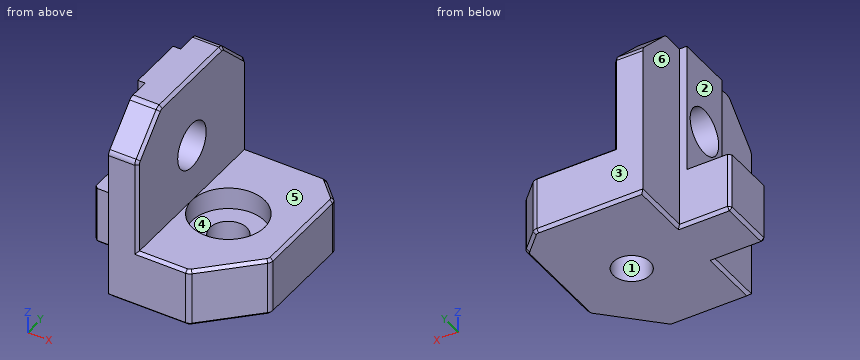
from build123d import *

# Parameters (mm, degrees)
CYLINDER014_R     = 3.15
CYLINDER014_DEPTH = 15
BOX016_W          = 4
BOX016_H          = 24
BOX016_DEPTH      = 26
CHAMFER024_SIZE   = 5
FILLET006_R       = 1
CHAMFER025_SIZE   = 0.4
CYLINDER012_R     = 2.525
CYLINDER012_DEPTH = 35
CYLINDER013_R     = 5
CYLINDER013_DEPTH = 5
BOX018_W          = 18
BOX018_H          = 24
BOX018_DEPTH      = 8
CHAMFER021_SIZE   = 7
CHAMFER022_SIZE   = 3
FILLET005_R       = 1
CHAMFER023_SIZE   = 0.4
BOX019_W          = 2
BOX019_H          = 7.8
BOX019_DEPTH      = 18
BOX017_W          = 8
BOX017_H          = 7.8
BOX017_DEPTH      = 8
CHAMFER026_SIZE   = 0.4


with BuildPart() as cylinder014:
    # Cylinder014 → Cylinder014 (new body)
    with BuildSketch(Plane(origin=(9, 15, 56), x_dir=(0, -1, 0), z_dir=(-1, 0, 0))):
        Circle(CYLINDER014_R)
    extrude(amount=CYLINDER014_DEPTH)


with BuildPart() as chamfer025:
    # Box016 → Box016 (new body)
    with BuildSketch(Plane(origin=(0, 3, 40), x_dir=(1, 0, 0), z_dir=(0, 0, 1))):
        with Locations((2, 12)):
            Rectangle(BOX016_W, BOX016_H)
    extrude(amount=BOX016_DEPTH)

    # Chamfer024
    chamfer024_edges = [chamfer025.edges().sort_by_distance(p)[0] for p in [
        (2, 3, 66),
        (2, 27, 66),
    ]]
    chamfer(chamfer024_edges, length=CHAMFER024_SIZE)

    # Fillet006
    fillet006_edges = [chamfer025.edges().sort_by_distance(p)[0] for p in [
        (2, 3, 61),
        (2, 8, 66),
        (2, 22, 66),
        (2, 27, 61),
    ]]
    fillet(fillet006_edges, radius=FILLET006_R)

    # Chamfer025
    chamfer025_edges = [chamfer025.edges().sort_by_distance(p)[0] for p in [
        (0, 15, 40),
        (4, 3, 50.292893),
        (2, 3, 40),
        (4, 3.07612, 60.96847),
        (2, 27, 40),
        (4, 15, 40),
        (4, 5.5, 63.5),
        (4, 27, 50.292893),
        (4, 8.03153, 65.92388),
        (4, 26.92388, 60.96847),
        (4, 15, 66),
        (4, 24.5, 63.5),
        (4, 21.96847, 65.92388),
    ]]
    chamfer(chamfer025_edges, length=CHAMFER025_SIZE)


with BuildPart() as cylinder012:
    # Cylinder012 → Cylinder012 (new body)
    with BuildSketch(Plane(origin=(9, 15, 32.7), x_dir=(1, 0, 0), z_dir=(0, 0, 1))):
        Circle(CYLINDER012_R)
    extrude(amount=CYLINDER012_DEPTH)


with BuildPart() as cylinder013:
    # Cylinder013 → Cylinder013 (new body)
    with BuildSketch(Plane(origin=(9, 15, 45), x_dir=(1, 0, 0), z_dir=(0, 0, 1))):
        Circle(CYLINDER013_R)
    extrude(amount=CYLINDER013_DEPTH)


with BuildPart() as cut002002002007004003:
    # Box018 → Box018 (new body)
    with BuildSketch(Plane(origin=(0, 3, 40), x_dir=(1, 0, 0), z_dir=(0, 0, 1))):
        with Locations((9, 12)):
            Rectangle(BOX018_W, BOX018_H)
    extrude(amount=BOX018_DEPTH)

    # Chamfer021
    chamfer021_edges = [cut002002002007004003.edges().sort_by_distance(p)[0] for p in [
        (18, 3, 44),
    ]]
    chamfer(chamfer021_edges, length=CHAMFER021_SIZE)

    # Chamfer022
    chamfer022_edges = [cut002002002007004003.edges().sort_by_distance(p)[0] for p in [
        (18, 27, 44),
    ]]
    chamfer(chamfer022_edges, length=CHAMFER022_SIZE)

    # Fillet005
    fillet005_edges = [cut002002002007004003.edges().sort_by_distance(p)[0] for p in [
        (18, 10, 44),
        (18, 24, 44),
        (15, 27, 44),
        (11, 3, 44),
    ]]
    fillet(fillet005_edges, radius=FILLET005_R)

    # Chamfer023
    chamfer023_edges = [cut002002002007004003.edges().sort_by_distance(p)[0] for p in [
        (18, 17, 48),
        (18, 17, 40),
        (17.92388, 23.96847, 48),
        (16.5, 25.5, 48),
        (14.96847, 26.92388, 48),
        (7.292893, 27, 48),
        (0, 15, 48),
        (5.292893, 3, 48),
        (10.96847, 3.07612, 48),
        (14.5, 6.5, 48),
        (17.92388, 10.03153, 48),
        (17.92388, 10.03153, 40),
        (17.92388, 23.96847, 40),
        (16.5, 25.5, 40),
        (14.96847, 26.92388, 40),
        (7.292893, 27, 40),
        (0, 15, 40),
        (5.292893, 3, 40),
        (10.96847, 3.07612, 40),
        (14.5, 6.5, 40),
    ]]
    chamfer(chamfer023_edges, length=CHAMFER023_SIZE)

    # Cut002002002007004002: cut Cylinder013
    add(cylinder013.part, mode=Mode.SUBTRACT)

    # Cut002002002007004003: cut Cylinder012
    add(cylinder012.part, mode=Mode.SUBTRACT)


with BuildPart() as cube019:
    # Box019 → Box019 (new body)
    with BuildSketch(Plane(origin=(-1, 11.1, 48), x_dir=(1, 0, 0), z_dir=(0, 0, 1))):
        with Locations((1, 3.9)):
            Rectangle(BOX019_W, BOX019_H)
    extrude(amount=BOX019_DEPTH)


with BuildPart() as obj1:
    # Box017 → Box017 (new body)
    with BuildSketch(Plane(origin=(-7, 11.1, 40), x_dir=(1, 0, 0), z_dir=(0, 0, 1))):
        with Locations((4, 3.9)):
            Rectangle(BOX017_W, BOX017_H)
    extrude(amount=BOX017_DEPTH)

    # Chamfer026
    chamfer026_edges = [obj1.edges().sort_by_distance(p)[0] for p in [
        (-7, 11.1, 44),
        (-7, 18.9, 44),
        (-7, 15, 40),
        (-3, 11.1, 40),
        (-3, 18.9, 40),
    ]]
    chamfer(chamfer026_edges, length=CHAMFER026_SIZE)

    # Fusion006005: union Chamfer025, Cut002002002007004003, Cube019
    add(chamfer025.part)
    add(cut002002002007004003.part)
    add(cube019.part)

    # Cut002002002007004004: cut Cylinder014
    add(cylinder014.part, mode=Mode.SUBTRACT)


solid = obj1.part
Geometry: final body of the model. Coordinates: model frame, mm. Face numbers are marked on the shaded views. A direction names the side the tool comes from. Coordinates: 2 decimals unless noted, no trailing zeros. Order: outer loops, then holes, each group sorted by start corner. A loop starts at its lowest first (then second) coordinate and runs counter-clockwise, first axis right, second up.
(1) Material intervals for probe 1 along Z at (x, y) = (1.35, 15); probe 2 along X at (y, z) = (15, 45.8); probe 3 along Y at (x, z) = (9, 46.2), sorted ascending.
(2) Section query A-A (x = 9). Return the cut outline in (y, z) (3 decimals).
(3) Section query B-B (z = 56). Return the cut outline in (x, y).
(4) Draft query along X for the marked faces 1, 2 and 3. Return one class per face: pulls with the +X half, pulls with the -X half, needs draft (parallel to the pull), parting line crosses it, or undercut.
(5) Section query C-C (z = 46). Return the cut outline in (x, y).
(6) Access query for the marked faces 4, 5 and 6. Directions: +Z, -Z, +X, -X, +Y, -Y. A direction counts if a zero-diameter tool reaches every point of the face in a straight line with its end or side. Return the directions, or none.
(7) Section query D-D (x = 2). Return the cut outline in (y, z).
(8) First-contact query: pin 1 (6 mm diameter, centred on y = 14.5, z = 54, fed in from -X); pin 2 (5 mm diameter, centred on x = 8, y = 13.5, fed in from +Z); pin 3 (3.5 mm diameter, centred on x = -2, z = 54, fed in from -Y); pin 4 (4 mm diameter, centred on y = 15, z = 56, fed in from +X). Flat tips, straight axial feed; report the tip coordinate or a pass-through.
Solution:
1. probe 1: z = 40 to 52.85, 59.15 to 66
1. probe 2: x = -7 to 4, 14 to 18
1. probe 3: y = 3 to 10, 20 to 27
2. outline: (3, 40.4) - (3.4, 40) - (12.475, 40) - (12.475, 45) - (10, 45) - (10, 48) - (3.4, 48) - (3, 47.6) - close; (17.525, 40) - (26.6, 40) - (27, 40.4) - (27, 47.6) - (26.6, 48) - (20, 48) - (20, 45) - (17.525, 45) - close
3. outline: (-1, 11.1) - (0, 11.1) - (0, 3) - (3.6, 3) - (4, 3.4) - (4, 11.85) - (-1, 11.85) - close; (-1, 18.15) - (4, 18.15) - (4, 26.6) - (3.6, 27) - (0, 27) - (0, 18.9) - (-1, 18.9) - close
4. face 1: undercut
4. face 2: pulls with the -X half
4. face 3: needs draft
5. outline: (-7, 11.5) - (-6.6, 11.1) - (0, 11.1) - (0, 3) - (10.59, 3) arc R1 ccw to (11.29, 3.29) - (17.71, 9.71) arc R1 ccw to (18, 10.41) - (18, 23.59) arc R1 ccw to (17.71, 24.29) - (15.29, 26.71) arc R1 ccw to (14.59, 27) - (0, 27) - (0, 18.9) - (-6.6, 18.9) - (-7, 18.5) - close; hole circle Ø10 at (9, 15)
6. face 4: +Z
6. face 5: +Z, +X, +Y, -Y
6. face 6: +Z, -Z, -X, +Y
7. outline: (3, 40.4) - (3.4, 40) - (26.6, 40) - (27, 40.4) - (27, 60.59) arc R1 ccw to (26.71, 61.29) - (22.29, 65.71) arc R1 ccw to (21.59, 66) - (8.41, 66) arc R1 ccw to (7.71, 65.71) - (3.29, 61.29) arc R1 ccw to (3, 60.59) - close; hole circle Ø6.3 at (15, 56)
8. pin 1: stops at x = -1
8. pin 2: stops at z = 45
8. pin 3: stops at y = 11.1
8. pin 4: passes through
